```python
from build123d import *
from build123d.topology import SkipClean

# Parameters (mm, degrees)
SKETCH1_R           = 4.5
BOSS_EXTRUDE1_DEPTH = 1.5
BOSS_EXTRUDE2_DEPTH = 2
BOSS_EXTRUDE3_DEPTH = 6
BOSS_EXTRUDE4_DEPTH = 4.5


with BuildPart() as part:
    # Sketch1 → Boss-Extrude1 (new body)
    with BuildSketch(Plane(origin=(0, 0, 0), x_dir=(1, 0, 0), z_dir=(0, 1, 0))):
        with Locations(Location((0, 0, 0), (0, 0, 270))):
            Circle(SKETCH1_R)
    extrude(amount=BOSS_EXTRUDE1_DEPTH)

    # Sketch2 → Boss-Extrude2 (add)
    with SkipClean():  # the faces are left unmerged after this step: merging them gives an invalid solid
        with BuildSketch(Plane.XZ):
            with BuildLine():
                ThreePointArc((-1.152171862, 4.35), (-2.43566088, 3.783854658), (-3.48245603, 2.85))
                Line((-3.48245603, 2.85), (3.48245603, 2.85))
                ThreePointArc((3.48245603, 2.85), (2.43566088, 3.783854658), (1.152171862, 4.35))
                Line((1.152171862, 4.35), (-1.152171862, 4.35))
            make_face()
            with BuildLine():
                Line((-3.6, 1.5), (-4.242640687, 1.5))
                ThreePointArc((-4.242640687, 1.5), (-4.5, 0), (-4.242640687, -1.5))
                Line((-4.242640687, -1.5), (-3.6, -1.5))
                ThreePointArc((-3.6, -1.5), (-3.9, 0), (-3.6, 1.5))
            make_face()
            with BuildLine():
                Line((4.242640687, 1.5), (3.6, 1.5))
                ThreePointArc((3.6, 1.5), (3.9, 0), (3.6, -1.5))
                Line((3.6, -1.5), (4.242640687, -1.5))
                ThreePointArc((4.242640687, -1.5), (4.5, 0), (4.242640687, 1.5))
            make_face()
            with BuildLine():
                Line((3.48245603, -2.85), (-3.48245603, -2.85))
                ThreePointArc((-3.48245603, -2.85), (-2.43566088, -3.783854658), (-1.152171862, -4.35))
                Line((-1.152171862, -4.35), (1.152171862, -4.35))
                ThreePointArc((1.152171862, -4.35), (2.43566088, -3.783854658), (3.48245603, -2.85))
            make_face()
        extrude(amount=BOSS_EXTRUDE2_DEPTH)

    # Sketch3 → Boss-Extrude3 (add)
    with SkipClean():  # the faces are left unmerged after this step: merging them gives an invalid solid
        with BuildSketch(Plane.XZ.offset(2)):
            with BuildLine():
                ThreePointArc((-1.152171862, 4.35), (-2.43566088, 3.783854658), (-3.48245603, 2.85))
                Line((-3.48245603, 2.85), (3.48245603, 2.85))
                ThreePointArc((3.48245603, 2.85), (2.43566088, 3.783854658), (1.152171862, 4.35))
                Line((1.152171862, 4.35), (-1.152171862, 4.35))
            make_face()
            with BuildLine():
                Line((3.48245603, -2.85), (-3.48245603, -2.85))
                ThreePointArc((-3.48245603, -2.85), (-2.43566088, -3.783854658), (-1.152171862, -4.35))
                Line((-1.152171862, -4.35), (1.152171862, -4.35))
                ThreePointArc((1.152171862, -4.35), (2.43566088, -3.783854658), (3.48245603, -2.85))
            make_face()
        extrude(amount=BOSS_EXTRUDE3_DEPTH)

    # Sketch4 → Boss-Extrude4 (add)
    with SkipClean():  # the faces are left unmerged after this step: merging them gives an invalid solid
        with BuildSketch(Plane.XZ.offset(8)):
            with BuildLine():
                ThreePointArc((1.152171862, -4.35), (2.43566088, -3.783854658), (3.48245603, -2.85))
                Line((3.48245603, -2.85), (-3.48245603, -2.85))
                ThreePointArc((-3.48245603, -2.85), (-2.43566088, -3.783854658), (-1.152171862, -4.35))
                Line((-1.152171862, -4.35), (1.152171862, -4.35))
            make_face()
            with BuildLine():
                ThreePointArc((-4.102133591, -1.85), (-3.825114368, -2.370337543), (-3.48245603, -2.85))
                Line((-3.48245603, -2.85), (3.48245603, -2.85))
                ThreePointArc((3.48245603, -2.85), (3.825114368, -2.370337543), (4.102133591, -1.85))
                Line((4.102133591, -1.85), (-4.102133591, -1.85))
            make_face()
            with BuildLine():
                ThreePointArc((-1.152171862, 4.35), (-2.909369597, 3.433011586), (-4.102133591, 1.85))
                Line((-4.102133591, 1.85), (4.102133591, 1.85))
                ThreePointArc((4.102133591, 1.85), (2.909369597, 3.433011586), (1.152171862, 4.35))
                Line((1.152171862, 4.35), (-1.152171862, 4.35))
            make_face()
        extrude(amount=BOSS_EXTRUDE4_DEPTH)


solid = part.part
```
Part model, mm, in its own coordinate system. A direction names the side the tool comes from. Give positions to 0.01 mm unless a question says otherwise; leave off trailing zeros. Order: outer loops, then holes, each group sorted by start corner. A loop starts at its lowest first (then second) coordinate and runs counter-clockwise, first axis right, second up. Notation, with made-up numbers: M 16.5,-25 L 33.5,-25 A27 cw 33.5,12 Z; hole C 42,-23 d2. An arc over 180 degrees is marked long. Use a Markdown table: item, result. Add a question column.
(1) Probe line 1 along Z through (x, y) = (-0.75, -4.25); line 2 along Y through (x, z) = (3.75, 2). List the from-to ranges inside material, lowest first. Write a range as [from, to].
(2) Saw through at A-A, the plane y = -9.25. Give the cut face in (x, z), and give its area (3 significant figures).
(3) Saw through at D-D, the plane x = 3. Give the cut face in (y, z).
(4) Saw through at B-B, the plane z = 0. Give the cut face in (x, y), and give its area (3 significant figures).
(5) Saw through at C-C, the plane x = 0. Give the cut face in (y, z).
(6) 3-axis set-ups, long thin cutter, end or side, ignore diameter. For faces 1 (the face through (0, -6, -4.35)), 2 (the face through (-0.1, -8, 2.4)), 3 (the face through (0, -10, 1.85)): which of +Z, -Z, +X, -X, +Y, -Y reach the whole face in a straight line?
(7) Drop flat-ended pins along their axis: P1, Ø3.5, axis at x = 1, y = -4, coming from the -Z side; P2, Ø1, axis at x = 4, z = -0.5, coming from the -Y side; P3, Ø1.2, axis at x = 0.5, y = -6.5, coming from the +Z side. Give the stop position or say it passes through.
(8) Mould opens along Y. For faces 4 (the face through (0, 1.5, 0)), 5 (the face through (0, -4, 2.85)), 6 (the face through (0, -6, 4.35)) say: +Y half, -Y half, draft (parallel to the pull), parting line (faces both ways), or undercut.
Answer key:
| question | item | result |
|---|---|---|
| 1 | line 1 | [-4.35, -2.85], [2.85, 4.35] |
| 1 | line 2 | [-12.5, -8], [0, 1.5] |
| 2 | outline | M -4.1,-1.85 A4.5 ccw -1.15,-4.35 L 1.15,-4.35 A4.5 ccw 4.1,-1.85 Z; M -4.1,1.85 L 4.1,1.85 A4.5 ccw 1.15,4.35 L -1.15,4.35 A4.5 ccw Z |
| 2 | area | 30.8 mm^2 |
| 3 | outline | M -12.5,-3.35 L 1.5,-3.35 L 1.5,3.35 L -12.5,3.35 L -12.5,1.85 L -8,1.85 L -8,2.85 L 0,2.85 L 0,-2.85 L -8,-2.85 L -8,-1.85 L -12.5,-1.85 Z |
| 4 | outline | M -4.5,-2 L -3.9,-2 L -3.9,0 L 3.9,0 L 3.9,-2 L 4.5,-2 L 4.5,1.5 L -4.5,1.5 Z |
| 4 | area | 15.9 mm^2 |
| 5 | outline | M -12.5,-4.35 L 0,-4.35 L 0,-4.5 L 1.5,-4.5 L 1.5,4.5 L 0,4.5 L 0,4.35 L -12.5,4.35 L -12.5,1.85 L -8,1.85 L -8,2.85 L 0,2.85 L 0,-2.85 L -8,-2.85 L -8,-1.85 L -12.5,-1.85 Z |
| 6 | face 1 | -Z, +X, -X, -Y |
| 6 | face 2 | +X, -X |
| 6 | face 3 | +X, -X, -Y |
| 7 | P1 | z = -4.35 |
| 7 | P2 | y = -2 |
| 7 | P3 | z = 4.35 |
| 8 | face 4 | +Y half |
| 8 | face 5 | undercut |
| 8 | face 6 | draft |
